Can you work these out from the model? Positions are in its coordinate system, mm. A direction names the side the tool comes from. Coordinates: 2 decimals unless noted, no trailing zeros. Order: outer loops, then holes, each group sorted by start corner. A loop starts at its lowest first (then second) coordinate and runs counter-clockwise, first axis right, second up. Notation, with made-up numbers: (17, -39.75) -> (38, -39.75) arc R20 ccw to (38, -26.75) -> close; hole circle Ø9 at (61, 2). An arc over 180 degrees is marked (long way). Answer as a JSON object with one key per item and string values. Group by question number.
(1) I want a section at B-B, the plane x = -17.5. List the corners of the cut face in (y, z) for me.
(2) I want a section at C-C, the plane x = -8. List the corners of the cut face in (y, z) for me (3 decimals), plus the area to 3 significant figures.
(3) I want a section at D-D, the plane z = 1.1. State how many separate pieces and enclosed holes the cut face has, plus the area to 3 significant figures.
(4) If we mould it in two halves opening along X, with no side actions, what happens to faces 4 (the flat face through (-5, 16, 2)), 5 (the flat face through (16, 8, 1)), 6 (the flat face through (-10, 12, 0))? For each: pulls with the +X half, pulls with the -X half, needs draft (parallel to the pull), parting line crosses it, or undercut.
(5) Which directions (+Z, -Z, +X, -X, +Y, -Y) give clear straight access to the entire face, cutting with the end or side of a thin tool? Please do faces 1 (the flat face through (-11, 20, 1)), 2 (the flat face through (-5.5, 27, 2)), 3 (the cylindrical face through (11.57, 3.45, 1.52)).
(6) I need wall thicknesses on line 1 (Y direction, x = 1.5, z = 0.25); line 2 (X direction, y = 1.5, z = 0.75); line 3 (X direction, y = 17, z = 2.8). Which ranges of each line are inside material? Lowest first, please.
(7) I want a section at A-A, the plane y = 26. List the corners of the cut face in (x, z) for me (3 decimals), plus the area to 4 significant figures.
(8) For pin 1 (1.5 mm diameter, centred on y = 19, z = 2, fed in from +X); pin 2 (1.2 mm diameter, centred on y = 27, z = 1.5, fed in from +X); pin 3 (0.9 mm diameter, centred on x = -4.5, z = 1, fed in from +Y), each with a flat end and sliding along its axis, tell me the tip position at first contact or that it passes through.
from build123d import *

# Parameters (mm, degrees)
SKETCH1_R                = 0.5
BOSS_EXTRUDE1_DEPTH      = 3
M2_5X0_45_TAPPED_HOLE1_D = 2.05
SKETCH4_W                = 16.5
SKETCH4_H                = 4.5
CUT_EXTRUDE1_DEPTH       = 4
FILLET1_R                = 2
M3_CLEARANCE_HOLE1_D     = 3.4
M3_CLEARANCE_HOLE1_DEPTH = 3
FILLET2_R                = 2


with BuildPart() as part:
    # Sketch1 → Boss-Extrude1 (new body)
    with BuildSketch(Plane.XY):
        Polygon((-21, 0), (21, 0), (21, 6), (11, 10), (11, 30), (-11, 30), (-11, 10), (-21, 6), align=None)
        with Locations((-8, 26)):
            Circle(SKETCH1_R, mode=Mode.SUBTRACT)
        with Locations((8, 13)):
            Circle(SKETCH1_R, mode=Mode.SUBTRACT)
        with Locations((-17.5, 3)):
            Circle(SKETCH1_R, mode=Mode.SUBTRACT)
        with Locations((17.5, 3)):
            Circle(SKETCH1_R, mode=Mode.SUBTRACT)
    extrude(amount=BOSS_EXTRUDE1_DEPTH)

    # M2.5x0.45 Tapped Hole1 (through all)
    with Locations(Plane.XY.offset(3)):
        with Locations((-8, 26), (8, 13)):
            Hole(M2_5X0_45_TAPPED_HOLE1_D / 2)

    # Sketch4 → Cut-Extrude1 (cut, through all)
    with BuildSketch(Plane.XY.offset(3)):
        with Locations((2.75, 27.75)):
            Rectangle(SKETCH4_W, SKETCH4_H)
        with BuildLine():
            Line((-3.5, 22), (3.5, 22))
            ThreePointArc((3.5, 22), (4.560660172, 21.560660172), (5, 20.5))
            Line((5, 20.5), (5, 10.870483803))
            ThreePointArc((5, 10.870483803), (5.20263486, 10.117593576), (5.755791592, 9.56811909))
            Line((5.755791592, 9.56811909), (11.244208408, 6.43188091))
            ThreePointArc((11.244208408, 6.43188091), (11.79736514, 5.882406424), (12, 5.129516197))
            Line((12, 5.129516197), (12, 4.5))
            ThreePointArc((12, 4.5), (11.560660172, 3.439339828), (10.5, 3))
            Line((10.5, 3), (-10.5, 3))
            ThreePointArc((-10.5, 3), (-11.560660172, 3.439339828), (-12, 4.5))
            Line((-12, 4.5), (-12, 5.129516197))
            ThreePointArc((-12, 5.129516197), (-11.79736514, 5.882406424), (-11.244208408, 6.43188091))
            Line((-11.244208408, 6.43188091), (-5.755791592, 9.56811909))
            ThreePointArc((-5.755791592, 9.56811909), (-5.20263486, 10.117593576), (-5, 10.870483803))
            Line((-5, 10.870483803), (-5, 20.5))
            ThreePointArc((-5, 20.5), (-4.560660172, 21.560660172), (-3.5, 22))
        make_face()
    extrude(amount=-CUT_EXTRUDE1_DEPTH, mode=Mode.SUBTRACT)

    # Fillet1
    fillet1_edges = [part.edges().sort_by_distance(p)[0] for p in [
        (-21, 6, 1.5),
        (-11, 10, 1.5),
        (-11, 30, 1.5),
        (11, 10, 1.5),
        (21, 6, 1.5),
        (-5.5, 30, 1.5),
        (11, 25.5, 1.5),
    ]]
    fillet(fillet1_edges, radius=FILLET1_R)

    # M3 Clearance Hole1
    with Locations(Plane.XY.offset(3)):
        with Locations((-17.5, 3), (17.5, 3)):
            Hole(M3_CLEARANCE_HOLE1_D / 2, depth=M3_CLEARANCE_HOLE1_DEPTH)

    # Fillet2
    fillet2_edges = [part.edges().sort_by_distance(p)[0] for p in [
        (21, 0, 1.5),
        (-21, 0, 1.5),
    ]]
    fillet(fillet2_edges, radius=FILLET2_R)


solid = part.part
Computed values:
{
 "1": {"outline": "(0, 0) -> (1.3, 0) -> (1.3, 3) -> (0, 3) -> close; (4.7, 0) -> (7.4, 0) -> (7.4, 3) -> (4.7, 3) -> close"},
 "2": {"outline": "(0, 0) -> (3, 0) -> (3, 3) -> (0, 3) -> close; (8.286, 0) -> (24.975, 0) -> (24.975, 3) -> (8.286, 3) -> close; (27.025, 0) -> (30, 0) -> (30, 3) -> (27.025, 3) -> close", "area": "68.0 mm2"},
 "3": {"separate pieces": "1", "enclosed holes": "5", "area": "459 mm2"},
 "4": {"face 4": "undercut", "face 5": "pulls with the +X half", "face 6": "needs draft"},
 "5": {"face 1": "+Z, -Z, -X, +Y", "face 2": "+Z, -Z, +X, +Y", "face 3": "+Z, -Z"},
 "6": {"line 1": "y = 0 to 3, 22 to 25.5", "line 2": "x = -20.94 to -18.3, -16.7 to 16.7, 18.3 to 20.94", "line 3": "x = -11 to -5, 5 to 11"},
 "7": {"outline": "(-11, 0) -> (-9.025, 0) -> (-9.025, 3) -> (-11, 3) -> close; (-6.975, 0) -> (-5.5, 0) -> (-5.5, 3) -> (-6.975, 3) -> close", "area": "10.35 mm2"},
 "8": {"pin 1": "stops at x = 11", "pin 2": "stops at x = -5.5", "pin 3": "stops at y = 25.5"}
}
